Could you check a few things on this model? Use its own coordinates, in mm. Face numbers are marked on the shaded views. A direction names the side the tool comes from. Give positions to 0.01 mm unless a question says otherwise; leave off trailing zeros. Order: outer loops, then holes, each group sorted by start corner. A loop starts at its lowest first (then second) coordinate and runs counter-clockwise, first axis right, second up. Notation, with made-up numbers: M -23.5,-36.75 L -15.5,-36.75 A14 ccw -15.5,-31.75 Z; hole C 25,58 d2. An arc over 180 degrees is marked long. Use a Markdown table: item, result. Add a question column.
```python
from build123d import *

# Parameters (mm, degrees)
AUFSATZ_LINEAR_AUSTRAGEN1_DEPTH = 0.5
SKIZZE2_W                       = 2
SKIZZE2_H                       = 10.1
AUFSATZ_LINEAR_AUSTRAGEN2_DEPTH = 0.5
FASE1_SIZE                      = 0.5
FASE1_SIZE2                     = 1.37373871
SKIZZE3_W                       = 2
SKIZZE3_H                       = 10.1
AUFSATZ_LINEAR_AUSTRAGEN3_DEPTH = 0.5
FASE3_SIZE                      = 0.5
FASE3_SIZE2                     = 1.37373871
FASE4_SIZE                      = 0.5
FASE5_SIZE                      = 0.5
SKIZZE4_R                       = 0.25
SCHNITT_LINEAR_AUSTRAGEN1_DEPTH = 11.1


with BuildPart() as part:
    # Skizze1 → Aufsatz-Linear austragen1 (new body, symmetric)
    with BuildSketch(Plane.XY):
        Polygon((-2, 2.75), (-2, 7.35), (2, 7.35), (2, 2.75), (2.5, 2.75), (2.5, -2.75), (-2.5, -2.75), (-2.5, 2.75), align=None)
    extrude(amount=AUFSATZ_LINEAR_AUSTRAGEN1_DEPTH, both=True)

    # Skizze2 → Aufsatz-Linear austragen2 (add)
    with BuildSketch(Plane.XY.offset(0.5)):
        with Locations((0, 2.3)):
            Rectangle(SKIZZE2_W, SKIZZE2_H)
    extrude(amount=AUFSATZ_LINEAR_AUSTRAGEN2_DEPTH)

    # Fase1
    fase1_edges = [part.edges().sort_by_distance(p)[0] for p in [
        (0, 7.35, 1),
    ]]
    fase1_side = [part.faces().sort_by_distance(p)[0] for p in [
        (0, 7.35, 0.15),
    ]]
    chamfer(fase1_edges, length=FASE1_SIZE, length2=FASE1_SIZE2, reference=fase1_side[0])

    # Skizze3 → Aufsatz-Linear austragen3 (add)
    with BuildSketch(Plane(origin=(0, 0, -0.5), x_dir=(-1, 0, 0), z_dir=(0, 0, -1))):
        with Locations((0, 2.3)):
            Rectangle(SKIZZE3_W, SKIZZE3_H)
    extrude(amount=AUFSATZ_LINEAR_AUSTRAGEN3_DEPTH)

    # Fase3
    fase3_edges = [part.edges().sort_by_distance(p)[0] for p in [
        (0, 7.35, -1),
    ]]
    fase3_side = [part.faces().sort_by_distance(p)[0] for p in [
        (0, 7.35, -0.15),
    ]]
    chamfer(fase3_edges, length=FASE3_SIZE, length2=FASE3_SIZE2, reference=fase3_side[0])

    # Fase4
    fase4_edges = [part.edges().sort_by_distance(p)[0] for p in [
        (-2, 7.35, 0),
    ]]
    chamfer(fase4_edges, length=FASE4_SIZE)

    # Fase5
    fase5_edges = [part.edges().sort_by_distance(p)[0] for p in [
        (2, 7.35, 0),
    ]]
    chamfer(fase5_edges, length=FASE5_SIZE)

    # Skizze4 → Schnitt-Linear austragen1 (cut, through all)
    with BuildSketch(Plane(origin=(0, 7.35, 0), x_dir=(1, 0, 0), z_dir=(0, 1, 0))):
        Circle(SKIZZE4_R)
    extrude(amount=-SCHNITT_LINEAR_AUSTRAGEN1_DEPTH, mode=Mode.SUBTRACT)


solid = part.part
```
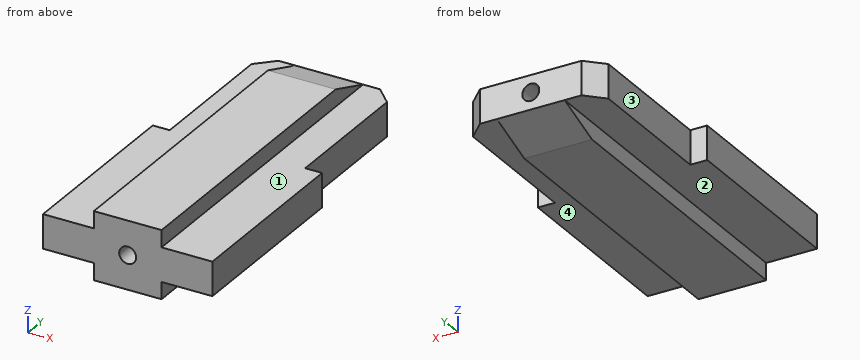
1) Suppose I cut it at B-B on z = 0. Please give me the cut outline in (x, y).
2) Please list where these lines run through material, in increasing order: line 1 (X direction, y = -1, z = 0); line 2 (Z direction, x = 0, y = 0.25); line 3 (X direction, y = 4.75, z = 0). Write a range as from..to.
3) Suppose I cut it at C-C on y = 6.25. Please give me the cut outline in (x, z), and give its area (3 significant figures).
4) Suppose I cut it at A-A on x = 0. Please give me the cut outline in (y, z), and give its area (3 significant figures).
5) For the marked faces 1, 2, 3 and 4, which set-ups out of +Z, -Z, +X, -X, +Y, -Y let a thin tool reach every point of the face, with its end or its side?
6) For pin 1 (1 mm diameter, centred on x = 2, y = 4.5, fed in from -Z); pin 2 (0.8 mm diameter, centred on x = -2, y = 2, fed in from +Z); pin 3 (1.1 mm diameter, centred on y = 4, z = 0, fed in from -X), each with a flat end and sliding along its axis, tell me the tip position at first contact or that it passes through.
7) Suppose I cut it at D-D on x = 0.75. Please give me the cut outline in (y, z), and give its area (3 significant figures).
Values found:
| question | item | result |
|---|---|---|
| 1 | outline | M -2.5,-2.75 L -0.25,-2.75 L -0.25,7.35 L -1.5,7.35 L -2,6.85 L -2,2.75 L -2.5,2.75 Z; M 0.25,-2.75 L 2.5,-2.75 L 2.5,2.75 L 2,2.75 L 2,6.85 L 1.5,7.35 L 0.25,7.35 Z |
| 2 | line 1 | x = -2.5..-0.25, 0.25..2.5 |
| 2 | line 2 | z = -1..-0.25, 0.25..1 |
| 2 | line 3 | x = -2..-0.25, 0.25..2 |
| 3 | outline | M -2,-0.5 L -1,-0.5 L -1,-0.9 L 1,-0.9 L 1,-0.5 L 2,-0.5 L 2,0.5 L 1,0.5 L 1,0.9 L -1,0.9 L -1,0.5 L -2,0.5 Z; hole C 0,0 d0.5 |
| 3 | area | 5.41 mm^2 |
| 4 | outline | M -2.75,-1 L 5.98,-1 L 7.35,-0.5 L 7.35,-0.25 L -2.75,-0.25 Z; M -2.75,0.25 L 7.35,0.25 L 7.35,0.5 L 5.98,1 L -2.75,1 Z |
| 4 | area | 14.5 mm^2 |
| 5 | face 1 | +Z, +X, +Y, -Y |
| 5 | face 2 | -Z, -X, +Y, -Y |
| 5 | face 3 | +Z, -Z, -X, +Y |
| 5 | face 4 | -Z, +X, +Y, -Y |
| 6 | pin 1 | stops at z = -0.5 |
| 6 | pin 2 | stops at z = 0.5 |
| 6 | pin 3 | stops at x = -2 |
| 7 | outline | M -2.75,-1 L 5.98,-1 L 7.35,-0.5 L 7.35,0.5 L 5.98,1 L -2.75,1 Z |
| 7 | area | 19.5 mm^2 |
